Model file for the job. Use its own axes, mm. A direction names the side the tool comes from. Coordinates: 2 decimals unless noted, no trailing zeros. Loops run counter-clockwise (first coordinate to the right, second up) from the corner with the lowest first, then second, coordinate; pieces in that order, holes last. Notation, with made-up numbers: (-31.75, 16) - (-8.75, 16) arc R19 cw to (-8.75, 26) - close; hole circle Ø3 at (36, 59). An arc over 180 degrees is marked (long way). Write each question's results on one line, items separated by ' | '. Start each with the question number.
```python
from build123d import *

# Parameters (mm, degrees)
SKETCH1_R           = 1.5
BOSS_EXTRUDE1_DEPTH = 6.35


with BuildPart() as part:
    # Sketch1 → Boss-Extrude1 (new body)
    with BuildSketch(Plane(origin=(0, 0, 0), x_dir=(-1, 0, 0), z_dir=(0, 0, -1))):
        with BuildLine():
            Line((151.502577388, 25), (-151.502577388, 25))
            ThreePointArc((-151.502577388, 25), (-153.002577388, 25.401923789), (-154.1006536, 26.5))
            ThreePointArc((-154.1006536, 26.5), (-156.391647728, 30.121613703), (-158.967745468, 33.54629768))
            ThreePointArc((-158.967745468, 33.54629768), (-159.465036881, 34.421268405), (-159.644975992, 35.411467596))
            ThreePointArc((-159.644975992, 35.411467596), (-161.109127035, 38.890872965), (-164.588532404, 40.355024008))
            ThreePointArc((-164.588532404, 40.355024008), (-165.578731594, 40.534963119), (-166.45370232, 41.032254532))
            ThreePointArc((-166.45370232, 41.032254532), (-200, 53), (-233.54629768, 41.032254532))
            ThreePointArc((-233.54629768, 41.032254532), (-234.421268405, 40.534963119), (-235.411467596, 40.355024008))
            ThreePointArc((-235.411467596, 40.355024008), (-238.890872965, 38.890872965), (-240.355024008, 35.411467596))
            ThreePointArc((-240.355024008, 35.411467596), (-240.534963119, 34.421268406), (-241.032254532, 33.54629768))
            ThreePointArc((-241.032254532, 33.54629768), (-253, 0), (-241.032254532, -33.54629768))
            ThreePointArc((-241.032254532, -33.54629768), (-240.534963119, -34.421268405), (-240.355024008, -35.411467596))
            ThreePointArc((-240.355024008, -35.411467596), (-238.890872965, -38.890872965), (-235.411467596, -40.355024008))
            ThreePointArc((-235.411467596, -40.355024008), (-234.421268406, -40.534963119), (-233.54629768, -41.032254532))
            ThreePointArc((-233.54629768, -41.032254532), (-200, -53), (-166.45370232, -41.032254532))
            ThreePointArc((-166.45370232, -41.032254532), (-165.578731595, -40.534963119), (-164.588532404, -40.355024008))
            ThreePointArc((-164.588532404, -40.355024008), (-161.109127035, -38.890872965), (-159.644975992, -35.411467596))
            ThreePointArc((-159.644975992, -35.411467596), (-159.465036881, -34.421268405), (-158.967745468, -33.54629768))
            ThreePointArc((-158.967745468, -33.54629768), (-156.391647728, -30.121613703), (-154.1006536, -26.5))
            ThreePointArc((-154.1006536, -26.5), (-153.002577388, -25.401923789), (-151.502577388, -25))
            Line((-151.502577388, -25), (151.502577388, -25))
            ThreePointArc((151.502577388, -25), (153.002577388, -25.401923789), (154.100653599, -26.5))
            ThreePointArc((154.100653599, -26.5), (156.391647728, -30.121613703), (158.967745468, -33.54629768))
            ThreePointArc((158.967745468, -33.54629768), (159.465036881, -34.421268405), (159.644975992, -35.411467596))
            ThreePointArc((159.644975992, -35.411467596), (161.109127035, -38.890872965), (164.588532404, -40.355024008))
            ThreePointArc((164.588532404, -40.355024008), (165.578731594, -40.534963119), (166.45370232, -41.032254532))
            ThreePointArc((166.45370232, -41.032254532), (200, -53), (233.546297679, -41.032254532))
            ThreePointArc((233.546297679, -41.032254532), (234.421268405, -40.534963119), (235.411467596, -40.355024008))
            ThreePointArc((235.411467596, -40.355024008), (238.890872965, -38.890872965), (240.355024008, -35.411467596))
            ThreePointArc((240.355024008, -35.411467596), (240.534963119, -34.421268405), (241.032254532, -33.546297679))
            ThreePointArc((241.032254532, -33.546297679), (253, 0), (241.032254532, 33.54629768))
            ThreePointArc((241.032254532, 33.54629768), (240.534963119, 34.421268406), (240.355024008, 35.411467596))
            ThreePointArc((240.355024008, 35.411467596), (238.890872965, 38.890872965), (235.411467596, 40.355024008))
            ThreePointArc((235.411467596, 40.355024008), (234.421268405, 40.534963119), (233.546297679, 41.032254532))
            ThreePointArc((233.546297679, 41.032254532), (200, 53), (166.45370232, 41.032254532))
            ThreePointArc((166.45370232, 41.032254532), (165.578731594, 40.534963119), (164.588532404, 40.355024008))
            ThreePointArc((164.588532404, 40.355024008), (161.109127035, 38.890872965), (159.644975992, 35.411467596))
            ThreePointArc((159.644975992, 35.411467596), (159.465036881, 34.421268406), (158.967745468, 33.54629768))
            ThreePointArc((158.967745468, 33.54629768), (156.391647727, 30.121613703), (154.100653599, 26.5))
            ThreePointArc((154.100653599, 26.5), (153.002577388, 25.401923789), (151.502577388, 25))
        make_face()
        with Locations((-235.355339059, -35.355339059)):
            Circle(SKETCH1_R, mode=Mode.SUBTRACT)
        with Locations((-235.355339059, 35.355339059)):
            Circle(SKETCH1_R, mode=Mode.SUBTRACT)
        with Locations((-164.644660941, -35.355339059)):
            Circle(SKETCH1_R, mode=Mode.SUBTRACT)
        with Locations((-164.644660941, 35.355339059)):
            Circle(SKETCH1_R, mode=Mode.SUBTRACT)
        with Locations((235.355339059, -35.355339059)):
            Circle(SKETCH1_R, mode=Mode.SUBTRACT)
        with Locations((235.355339059, 35.355339059)):
            Circle(SKETCH1_R, mode=Mode.SUBTRACT)
        with Locations((164.644660941, -35.355339059)):
            Circle(SKETCH1_R, mode=Mode.SUBTRACT)
        with Locations((164.644660941, 35.355339059)):
            Circle(SKETCH1_R, mode=Mode.SUBTRACT)
        with Locations((75, 13)):
            Circle(SKETCH1_R, mode=Mode.SUBTRACT)
        with Locations((75, -13)):
            Circle(SKETCH1_R, mode=Mode.SUBTRACT)
        with Locations((-75, -13)):
            Circle(SKETCH1_R, mode=Mode.SUBTRACT)
        with Locations((-75, 13)):
            Circle(SKETCH1_R, mode=Mode.SUBTRACT)
        with Locations((140, 13)):
            Circle(SKETCH1_R, mode=Mode.SUBTRACT)
        with Locations((140, -13)):
            Circle(SKETCH1_R, mode=Mode.SUBTRACT)
        with Locations((-140, -13)):
            Circle(SKETCH1_R, mode=Mode.SUBTRACT)
        with Locations((-140, 13)):
            Circle(SKETCH1_R, mode=Mode.SUBTRACT)
        with BuildLine():
            Line((136, 14), (136, -14))
            ThreePointArc((136, -14), (135.121320344, -16.121320344), (133, -17))
            Line((133, -17), (82, -17))
            ThreePointArc((82, -17), (79.878679656, -16.121320344), (79, -14))
            Line((79, -14), (79, 14))
            ThreePointArc((79, 14), (79.878679656, 16.121320344), (82, 17))
            Line((82, 17), (133, 17))
            ThreePointArc((133, 17), (135.121320344, 16.121320344), (136, 14))
        make_face(mode=Mode.SUBTRACT)
        with BuildLine():
            Line((71, 14), (71, -14))
            ThreePointArc((71, -14), (70.121320344, -16.121320344), (68, -17))
            Line((68, -17), (-68, -17))
            ThreePointArc((-68, -17), (-70.121320344, -16.121320344), (-71, -14))
            Line((-71, -14), (-71, 14))
            ThreePointArc((-71, 14), (-70.121320344, 16.121320344), (-68, 17))
            Line((-68, 17), (68, 17))
            ThreePointArc((68, 17), (70.121320344, 16.121320344), (71, 14))
        make_face(mode=Mode.SUBTRACT)
        with BuildLine():
            Line((-136, -14), (-136, 14))
            ThreePointArc((-136, 14), (-135.121320344, 16.121320344), (-133, 17))
            Line((-133, 17), (-82, 17))
            ThreePointArc((-82, 17), (-79.878679656, 16.121320344), (-79, 14))
            Line((-79, 14), (-79, -14))
            ThreePointArc((-79, -14), (-79.878679656, -16.121320344), (-82, -17))
            Line((-82, -17), (-133, -17))
            ThreePointArc((-133, -17), (-135.121320344, -16.121320344), (-136, -14))
        make_face(mode=Mode.SUBTRACT)
        with BuildLine():
            ThreePointArc((-163.234137081, -29.279196093), (-164.12216388, -30.031781356), (-165.229806783, -30.389696669))
            ThreePointArc((-165.229806783, -30.389696669), (-168.180194847, -31.819805153), (-169.610303331, -34.770193217))
            ThreePointArc((-169.610303331, -34.770193217), (-169.968218644, -35.87783612), (-170.720803907, -36.765862919))
            ThreePointArc((-170.720803907, -36.765862919), (-200, -47), (-229.279196093, -36.765862918))
            ThreePointArc((-229.279196093, -36.765862918), (-230.031781356, -35.87783612), (-230.38969667, -34.770193216))
            ThreePointArc((-230.38969667, -34.770193216), (-231.819805153, -31.819805153), (-234.770193217, -30.38969667))
            ThreePointArc((-234.770193217, -30.38969667), (-235.87783612, -30.031781356), (-236.765862918, -29.279196093))
            ThreePointArc((-236.765862918, -29.279196093), (-247, 0), (-236.765862918, 29.279196093))
            ThreePointArc((-236.765862918, 29.279196093), (-235.87783612, 30.031781356), (-234.770193216, 30.38969667))
            ThreePointArc((-234.770193216, 30.38969667), (-231.819805153, 31.819805153), (-230.38969667, 34.770193217))
            ThreePointArc((-230.38969667, 34.770193217), (-230.031781356, 35.87783612), (-229.279196093, 36.765862918))
            ThreePointArc((-229.279196093, 36.765862918), (-200, 47), (-170.720803907, 36.765862918))
            ThreePointArc((-170.720803907, 36.765862918), (-169.968218644, 35.87783612), (-169.61030333, 34.770193216))
            ThreePointArc((-169.61030333, 34.770193216), (-168.180194847, 31.819805153), (-165.229806783, 30.38969667))
            ThreePointArc((-165.229806783, 30.38969667), (-164.12216388, 30.031781356), (-163.234137082, 29.279196093))
            ThreePointArc((-163.234137082, 29.279196093), (-153, 0), (-163.234137081, -29.279196093))
        make_face(mode=Mode.SUBTRACT)
        with BuildLine():
            ThreePointArc((165.229806783, -30.389696669), (164.12216388, -30.031781356), (163.234137081, -29.279196093))
            ThreePointArc((163.234137081, -29.279196093), (153, 0), (163.234137082, 29.279196093))
            ThreePointArc((163.234137082, 29.279196093), (164.12216388, 30.031781357), (165.229806783, 30.38969667))
            ThreePointArc((165.229806783, 30.38969667), (168.180194847, 31.819805154), (169.61030333, 34.770193217))
            ThreePointArc((169.61030333, 34.770193217), (169.968218643, 35.87783612), (170.720803907, 36.765862918))
            ThreePointArc((170.720803907, 36.765862918), (200, 47), (229.279196093, 36.765862919))
            ThreePointArc((229.279196093, 36.765862919), (230.031781356, 35.87783612), (230.38969667, 34.770193217))
            ThreePointArc((230.38969667, 34.770193217), (231.819805153, 31.819805154), (234.770193216, 30.38969667))
            ThreePointArc((234.770193216, 30.38969667), (235.87783612, 30.031781357), (236.765862918, 29.279196093))
            ThreePointArc((236.765862918, 29.279196093), (247, 0), (236.765862918, -29.279196093))
            ThreePointArc((236.765862918, -29.279196093), (235.87783612, -30.031781356), (234.770193216, -30.389696669))
            ThreePointArc((234.770193216, -30.389696669), (231.819805153, -31.819805153), (230.389696669, -34.770193216))
            ThreePointArc((230.389696669, -34.770193216), (230.031781356, -35.87783612), (229.279196093, -36.765862918))
            ThreePointArc((229.279196093, -36.765862918), (200, -47), (170.720803907, -36.765862919))
            ThreePointArc((170.720803907, -36.765862919), (169.968218644, -35.87783612), (169.610303331, -34.770193216))
            ThreePointArc((169.610303331, -34.770193216), (168.180194847, -31.819805153), (165.229806783, -30.389696669))
        make_face(mode=Mode.SUBTRACT)
    extrude(amount=-BOSS_EXTRUDE1_DEPTH)


solid = part.part
```
Q1. Cut at C-C (x = -201). List the corners of the cut face in (y, z), and give its area (3 significant figures).
Q2. Pin check, flat tips, straight feed: pin 1 (1.9 mm diameter, centred on x = 64, z = 2.5, fed in from +Y); pin 2 (3 mm diameter, centred on y = 5.5, z = 3, fed in from -X); pin 3 (3.5 mm diameter, centred on x = -235.36, y = 35.36, fed in from +Z); pin 4 (1.5 mm diameter, centred on y = -34, z = 2.5, fed in from -X). Stop position of each tip, or through.
Q3. Cut at B-B (y = -4.5). List the corners of the cut face in (x, z).
Q4. Which spindle directions (+Z, -Z, +X, -X, +Y, -Y) get a long thin tool onto all of the face, cutting with end or side? Do faces 4 (the cylindrical face through (247, 0, 3)), 5 (the cylindrical face through (-199.491, -52.998, 3.131)). Say none if no direction does.
Q5. Cut at A-A (x = 29). List the corners of the cut face in (y, z), and give its area (3 significant figures).
Q6. Drill centre lines: L1, parallel to Y at x = 140, z = 5.25; L2, parallel to Y at x = -4, z = 4.5; L3, parallel to X at y = 37, z = 4. Where is each one in solid material? Low to high. Write a range as from..to.
Q7. Mould opens along X. For faces 1 (the cylindrical face through (-252.998, -0.509, 3.131)), 2 (the cylindrical face through (-200.509, 52.998, 3.131)), 3 (the flat face through (1, -19, 6.35)) say: +X half, -X half, draft (parallel to the pull), parting line (faces both ways), or undercut.
Q8. Cut at D-D (z = 4). State how many separate pieces and enclosed holes the cut face has, and give its area (3 significant figures).
Check result:
1) outline: (-52.99, 0) - (-46.99, 0) - (-46.99, 6.35) - (-52.99, 6.35) - close; (46.99, 0) - (52.99, 0) - (52.99, 6.35) - (46.99, 6.35) - close | area: 76.2 mm²
2) pin 1: y = 25 | pin 2: x = -252.85 | pin 3: z = 6.35 | pin 4: x = -241.27
3) outline: (-252.81, 0) - (-246.78, 0) - (-246.78, 6.35) - (-252.81, 6.35) - close; (-153.22, 0) - (-136, 0) - (-136, 6.35) - (-153.22, 6.35) - close; (-79, 0) - (-71, 0) - (-71, 6.35) - (-79, 6.35) - close; (71, 0) - (79, 0) - (79, 6.35) - (71, 6.35) - close; (136, 0) - (153.22, 0) - (153.22, 6.35) - (136, 6.35) - close; (246.78, 0) - (252.81, 0) - (252.81, 6.35) - (246.78, 6.35) - close
4) face 4: +Z, -Z | face 5: +Z, -Z, -Y
5) outline: (-25, 0) - (-17, 0) - (-17, 6.35) - (-25, 6.35) - close; (17, 0) - (25, 0) - (25, 6.35) - (17, 6.35) - close | area: 102 mm²
6) L1: -25..-14.5, -11.5..11.5, 14.5..25 | L2: -25..-17, 17..25 | L3: -240.08..-228.98, -171.02..-159.92, 159.92..171.02, 228.98..240.08
7) face 1: -X half | face 2: undercut | face 3: draft
8) separate pieces: 1 | enclosed holes: 21 | area: 10,100 mm²
